Geometry check sheet. Reference: the model listing, model coordinates, mm. A direction names the side the tool comes from. Give positions to 0.01 mm unless a question says otherwise; leave off trailing zeros. Write each loop counter-clockwise with the first axis right and the second up, starting at its lowest first coordinate (ties: lowest second). Pieces come first, ordered by that corner, then holes. Notation, with made-up numbers: (16.25, 84) - (62.25, 84) arc R20 ccw to (62.25, 121) - close; hole circle Ø4 at (-14.5, 56.5). An arc over 180 degrees is marked (long way). Write item = value, one per line. Start each with the question number.
(1) Thickness scan on L1, parallel to X at y = 2, z = 0.45; L2, parallel to Y at x = 0, z = 0.35; L3, parallel to Y at x = -9, z = 1.6. Record the ranges inside material, lowest first.
(2) Section check B-B, the plane z = 2.5. Enter the section's corners in (x, y).
(3) Depth check by flat-ended pin: pin 1 Ø1.5 at (y, z) = (-10, 1) entering from -X; pin 2 Ø0.9 at (x, z) = (10, 2) entering from +Y. Enter the tip coordinate at first touch or a pass-through.
(4) Draft check along X on faces 4 (the flat face through (-4.345, 0, 2)), 5 (the flat face through (9, 7, 2)), 6 (the cylindrical face through (0.1, -13.54, 1.52)), 7 (the flat face through (8, -12, 1)). Enter one of: pulls with the +X half, pulls with the -X half, needs draft (parallel to the pull), parting line crosses it, or undercut.
(5) Section check C-C, the plane x = 0. Enter the section's corners in (y, z).
(6) Section check A-A, the plane y = 0. Enter the section's corners in (x, z), plus the area to 3 significant figures.
(7) Access from +Z, -Z, +X, -X, +Y, -Y to the whole of each face (thin tool, end or side, straight path). Record for faces 1 (the flat face through (-10, -7, 2)), 2 (the flat face through (4.345, 0, 2)), 3 (the flat face through (-8, 12, 1)).
```python
from build123d import *

# Parameters (mm, degrees)
SKETCH1_W           = 16
SKETCH1_H           = 33
BOSS_EXTRUDE1_DEPTH = 3
SKETCH2_W           = 22
SKETCH2_H           = 14
BOSS_EXTRUDE2_DEPTH = 3
CUT_EXTRUDE1_DEPTH  = 10


with BuildPart() as part:
    # Sketch1 → Boss-Extrude1 (new body)
    with BuildSketch(Plane.XY):
        Rectangle(SKETCH1_W, SKETCH1_H)
    extrude(amount=BOSS_EXTRUDE1_DEPTH)

    # Sketch2 → Boss-Extrude2 (add)
    with BuildSketch(Plane.XY.offset(3)):
        Rectangle(SKETCH2_W, SKETCH2_H)
    extrude(amount=-BOSS_EXTRUDE2_DEPTH)

    # Sketch3 → Cut-Extrude1 (cut)
    with BuildSketch(Plane.XY.offset(3)):
        with BuildLine():
            Line((4.345494921, 9.196065885), (4.345494921, -9.196065885))
            ThreePointArc((4.345494921, -9.196065885), (0, -13.541560806), (-4.345494921, -9.196065885))
            Line((-4.345494921, -9.196065885), (-4.345494921, 9.196065885))
            ThreePointArc((-4.345494921, 9.196065885), (0, 13.541560806), (4.345494921, 9.196065885))
        make_face()
    extrude(amount=-CUT_EXTRUDE1_DEPTH, mode=Mode.SUBTRACT)


solid = part.part
```
Model answer:
q1.L1 = -11 to -4.35, 4.35 to 11
q1.L2 = -16.5 to -13.54, 13.54 to 16.5
q1.L3 = -7 to 7
q2.outline = (-11, -7) - (-8, -7) - (-8, -16.5) - (8, -16.5) - (8, -7) - (11, -7) - (11, 7) - (8, 7) - (8, 16.5) - (-8, 16.5) - (-8, 7) - (-11, 7) - close; hole (-4.35, -9.2) arc R4.35 ccw to (4.35, -9.2) - (4.35, 9.2) arc R4.35 ccw to (-4.35, 9.2) - close
q3.pin_1 = -8
q3.pin_2 = 7
q4.face_4 = undercut
q4.face_5 = needs draft
q4.face_6 = undercut
q4.face_7 = pulls with the +X half
q5.outline = (-16.5, 0) - (-13.54, 0) - (-13.54, 3) - (-16.5, 3) - close; (13.54, 0) - (16.5, 0) - (16.5, 3) - (13.54, 3) - close
q6.outline = (-11, 0) - (-4.35, 0) - (-4.35, 3) - (-11, 3) - close; (4.35, 0) - (11, 0) - (11, 3) - (4.35, 3) - close
q6.area = 39.9 mm²
q7.face_1 = +Z, -Z, -X, -Y
q7.face_2 = +Z, -Z
q7.face_3 = +Z, -Z, -X, +Y
